Work out the finished part from the listing and answer in its coordinate system (mm). Coordinates: 2 decimals unless noted, no trailing zeros. Order: outer loops, then holes, each group sorted by start corner. A loop starts at its lowest first (then second) coordinate and runs counter-clockwise, first axis right, second up.
1. The part is cut by section B-B, the plane x = -30.5. Give the vertices of the cut face in (y, z), then the cut area to 3 significant figures.
2. The part is cut by section A-A, the plane y = 5. Give the vertices of the cut face in (x, z), then the cut area to 3 significant figures.
3. The part is cut by section C-C, the plane z = 1.65. Count the separate pieces of the cut face and the enclosed holes in it, then the cut area to 3 significant figures.
4. The part is cut by section D-D, the plane y = 24. Give the vertices of the cut face in (x, z), then the cut area to 3 significant figures.
5. Flat-ended cylindrical pins translate along their axes: pin 1 Ø2.5 at (x, y) = (-15.17, 2.5) entering from -Z; pin 2 Ø0.6 at (y, z) = (-24, 0.5) entering from -X; pin 3 Ø0.6 at (x, z) = (27.5, 1) entering from -Y. Find the tip coordinate at first contact, or state that the pin passes through.
6. Find the intervals of material crossed by probe 1 along Y at (x, z) = (-35.5, 0.55); probe 2 along X at (y, z) = (23, 1.2); probe 3 along X at (y, z) = (4.5, 0.35), in increasing order.
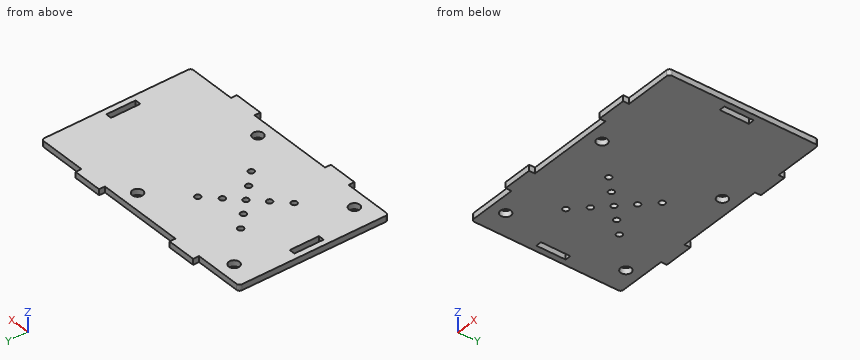
Solid Edge part; units mm, degrees
sketch "Sketch1" plane through (0, 0, 0) normal (0, 0, 1) x (1, 0, 0)
  line L0 (40, -25) -> (40, 30)
  line L1 (40, 30) -> (-44, 30)
  line L2 (-44, 30) -> (-44, -25)
  line L3 (-44, -25) -> (40, -25)
extrude "Protrusion1" add sketch "Sketch1" along normal blind 2
sketch "Sketch2" plane through (0, 0, 0) normal (0, 0, 1) x (1, 0, 0)
  line L0 (-44, 28) -> (-27, 28)
  line L1 (-27, 28) -> (-27, 30)
  line L2 (-27, 30) -> (-44, 30)
  line L3 (-44, 30) -> (-44, 28)
extrude "ExtrudedCutout_1" cut sketch "Sketch2" along normal blind 2
sketch "Sketch3" plane through (0, 0, 0) normal (0, 0, 1) x (1, 0, 0)
  line L0 (-17, 28) -> (13, 28)
  line L1 (13, 28) -> (13, 30)
  line L2 (13, 30) -> (-17, 30)
  line L3 (-17, 30) -> (-17, 28)
extrude "ExtrudedCutout_2" cut sketch "Sketch3" along normal blind 2
sketch "Sketch4" plane through (0, 0, 0) normal (0, 0, 1) x (1, 0, 0)
  line L0 (23, 28) -> (40, 28)
  line L1 (40, 28) -> (40, 30)
  line L2 (40, 30) -> (23, 30)
  line L3 (23, 30) -> (23, 28)
extrude "ExtrudedCutout_3" cut sketch "Sketch4" along normal blind 2
sketch "Sketch5" plane through (0, 0, 0) normal (0, 0, 1) x (1, 0, 0)
  line L0 (38, -2.5) -> (38, 7.5)
  line L1 (38, 7.5) -> (36, 7.5)
  line L2 (36, 7.5) -> (36, -2.5)
  line L3 (36, -2.5) -> (38, -2.5)
extrude "ExtrudedCutout_4" cut sketch "Sketch5" along normal blind 2
sketch "Sketch6" plane through (0, 0, 0) normal (0, 0, 1) x (1, 0, 0)
  line L0 (40, -23) -> (23, -23)
  line L1 (23, -23) -> (23, -25)
  line L2 (23, -25) -> (40, -25)
  line L3 (40, -25) -> (40, -23)
extrude "ExtrudedCutout_5" cut sketch "Sketch6" along normal blind 2
sketch "Sketch7" plane through (0, 0, 0) normal (0, 0, 1) x (1, 0, 0)
  line L0 (13, -23) -> (-17, -23)
  line L1 (-17, -23) -> (-17, -25)
  line L2 (-17, -25) -> (13, -25)
  line L3 (13, -25) -> (13, -23)
extrude "ExtrudedCutout_6" cut sketch "Sketch7" along normal blind 2
sketch "Sketch8" plane through (0, 0, 0) normal (0, 0, 1) x (1, 0, 0)
  line L0 (-27, -23) -> (-44, -23)
  line L1 (-44, -23) -> (-44, -25)
  line L2 (-44, -25) -> (-27, -25)
  line L3 (-27, -25) -> (-27, -23)
extrude "ExtrudedCutout_7" cut sketch "Sketch8" along normal blind 2
sketch "Sketch9" plane through (0, 0, 0) normal (0, 0, 1) x (1, 0, 0)
  line L0 (-40, -2.5) -> (-40, 7.5)
  line L1 (-40, 7.5) -> (-42, 7.5)
  line L2 (-42, 7.5) -> (-42, -2.5)
  line L3 (-42, -2.5) -> (-40, -2.5)
extrude "ExtrudedCutout_8" cut sketch "Sketch9" along normal blind 2
sketch "Sketch10" plane through (0, 0, 0) normal (0, 0, 1) x (1, 0, 0)
  circle A0 centre (-35.6965, 23.0215) radius 1.8
extrude "Cutout1" cut sketch "Sketch10" along normal blind 2
sketch "Sketch11" plane through (0, 0, 0) normal (0, 0, 1) x (1, 0, 0)
  circle A0 centre (5.3589, 23.016) radius 1.8
extrude "ExtrudedCutout_10" cut sketch "Sketch11" along normal blind 2
sketch "Sketch12" plane through (0, 0, 0) normal (0, 0, 1) x (1, 0, 0)
  circle A0 centre (-35.7266, -17.9943) radius 1.8
extrude "ExtrudedCutout_11" cut sketch "Sketch12" along normal blind 2
sketch "Sketch13" plane through (0, 0, 0) normal (0, 0, 1) x (1, 0, 0)
  circle A0 centre (5.346, -18.0319) radius 1.8
extrude "ExtrudedCutout_12" cut sketch "Sketch13" along normal blind 2
sketch "Sketch14" plane through (0, 0, 0) normal (0, 0, 1) x (1, 0, 0)
  circle A0 centre (-24.2914, 11.6184) radius 1
  circle A1 centre (-19.6326, 6.9596) radius 1
  circle A2 centre (-15.1715, 2.4985) radius 1
  circle A3 centre (-10.7104, 6.9596) radius 1
  circle A4 centre (-6.0516, 11.6184) radius 1
  circle A5 centre (-10.7104, -1.9626) radius 1
  circle A6 centre (-6.0516, -6.6214) radius 1
  circle A7 centre (-19.6326, -1.9626) radius 1
  circle A8 centre (-24.2914, -6.6214) radius 1
extrude "ExtrudedCutout_13" cut sketch "Sketch14" along normal blind 2
fillet "Round_1" radius 1 4 edges at (-44, -23, 1) (40, -23, 1) (40, 28, 1) (-44, 28, 1)
properties material "Acrylic, high impact grade"
Geometry says:
1. outline: (-23, 0) - (28, 0) - (28, 2) - (-23, 2) - close
1. area: 102 mm2
2. outline: (-44, 0) - (-42, 0) - (-42, 2) - (-44, 2) - close; (-40, 0) - (36, 0) - (36, 2) - (-40, 2) - close; (38, 0) - (40, 0) - (40, 2) - (38, 2) - close
2. area: 160 mm2
3. separate pieces: 1
3. enclosed holes: 15
3. area: 4,250 mm2
4. outline: (-44, 0) - (-37.21, 0) - (-37.21, 2) - (-44, 2) - close; (-34.19, 0) - (3.85, 0) - (3.85, 2) - (-34.19, 2) - close; (6.87, 0) - (40, 0) - (40, 2) - (6.87, 2) - close
4. area: 156 mm2
5. pin 1: stops at z = 0
5. pin 2: stops at x = -27
5. pin 3: stops at y = -23
6. probe 1: y = -23 to -19.78, -16.21 to 21.23, 24.81 to 28
6. probe 2: x = -44 to -37.5, -33.9 to 3.56, 7.16 to 40
6. probe 3: x = -44 to -42, -40 to 36, 38 to 40
